Could you check a few things on this model? Use its own coordinates, in mm. Face numbers are marked on the shaded views. A direction names the side the tool comes from. Round coordinates to 2 decimals unless told otherwise and drop trailing zeros. Loops run counter-clockwise (first coordinate to the right, second up) from the corner with the lowest first, then second, coordinate; pieces in that order, holes last. Notation, with made-up numbers: M -25,-12.5 L -17,-12.5 A18 ccw -17,12.5 Z; hole C -25.5,79 d7. An arc over 180 degrees is marked long. Answer in a Markdown table with one row per item.
```python
from build123d import *

# Parameters (mm, degrees)
FILLET_1_R               = 4
CUT_EXTRUDE_3_DEPTH      = 6
PATTERN_CIRCULAR_2_COUNT = 6
SKETCH_5_W               = 18.3
SKETCH_5_H               = 8
CUT_EXTRUDE_4_DEPTH      = 20
SKETCH_6_R               = 6
CUT_EXTRUDE_5_DEPTH      = 146.688022843
SKETCH_7_R               = 6.6215
CUT_EXTRUDE_6_DEPTH      = 146.688022843


with BuildPart() as part:
    # Sketch 1 → Revolve 1 (revolve)
    with BuildSketch(Plane(origin=(0, 0, 0), x_dir=(1, 0, 0), z_dir=(0, 1, 0)), mode=Mode.PRIVATE) as revolve_1_sk:
        Polygon((15, 20), (30, 20), (30, 6), (70, 6), (70, 15), (100, 15), (100, -15), (70, -15), (70, -6), (30, -6), (30, -20), (15, -20), align=None)
    revolve(revolve_1_sk.sketch.rotate(Axis((0, 0, -20), (0, 0, 1)), 180), axis=Axis((0, 0, -20), (0, 0, 1)))

    # Fillet 1
    fillet_1_edges = [part.edges().sort_by_distance(p)[0] for p in [
        (30, 0, 6),
        (70, 0, 6),
        (70, 0, -6),
        (30, 0, -6),
    ]]
    fillet(fillet_1_edges, radius=FILLET_1_R)

    # Sketch 4 → Cut-Extrude 3 (cut, symmetric)
    with BuildSketch(Plane.XY):
        with BuildLine():
            Line((41.5692, 6), (55.9285, 6))
            ThreePointArc((55.9285, 6), (59.790137098, 7.823876746), (60.8345, 11.9649))
            ThreePointArc((60.8345, 11.9649), (53.693292616, 30.999275079), (40.779, 46.7004))
            ThreePointArc((40.779, 46.7004), (36.670623538, 47.866536224), (33.1603, 45.4342))
            Line((33.1603, 45.4342), (25.9807, 32.9996))
            ThreePointArc((25.9807, 32.9996), (25.354603735, 29.839289607), (26.7862, 26.9531))
            ThreePointArc((26.7862, 26.9531), (32.908684734, 18.999699449), (36.7356, 9.7209))
            ThreePointArc((36.7356, 9.7209), (38.519259186, 7.037974406), (41.5692, 6))
        make_face()
    cut_extrude_3 = extrude(amount=CUT_EXTRUDE_3_DEPTH, both=True, mode=Mode.SUBTRACT)

    # Pattern Circular 2: Cut-Extrude 3 ×6 about axis
    pattern_circular_2_axis = Axis((0, 0, 0), (0, 0, 1))
    for i in range(1, PATTERN_CIRCULAR_2_COUNT):
        add(cut_extrude_3.rotate(pattern_circular_2_axis, i * 360 / PATTERN_CIRCULAR_2_COUNT), mode=Mode.SUBTRACT)

    # Sketch 5 → Cut-Extrude 4 (cut, symmetric)
    with BuildSketch(Plane.XY):
        with Locations((9.15, 0)):
            Rectangle(SKETCH_5_W, SKETCH_5_H)
    extrude(amount=CUT_EXTRUDE_4_DEPTH, both=True, mode=Mode.SUBTRACT)

    # Sketch 6 → Cut-Extrude 5 (cut, through all)
    with BuildSketch(Plane.XY.offset(15)):
        with Locations((92, 0)):
            Circle(SKETCH_6_R)
    extrude(amount=-CUT_EXTRUDE_5_DEPTH, mode=Mode.SUBTRACT)

    # Sketch 7 → Cut-Extrude 6 (cut, through all)
    with BuildSketch(Plane.XY.offset(15)):
        with Locations((-80, 0)):
            Circle(SKETCH_7_R)
    extrude(amount=-CUT_EXTRUDE_6_DEPTH, mode=Mode.SUBTRACT)


solid = part.part
```
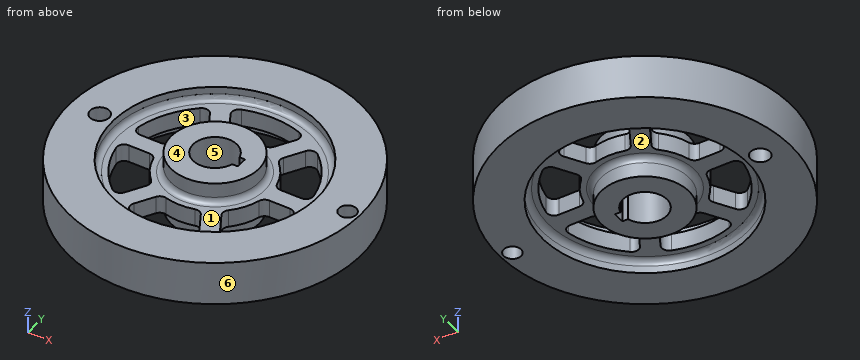
1) I want a section at A-A, the plane x = -80. Please give me the cut outline in (y, z).
Computed:
| item | result |
|---|---|
| outline | M -60,-15 L -6.62,-15 L -6.62,15 L -60,15 Z; M 6.62,-15 L 60,-15 L 60,15 L 6.62,15 Z |
2) Will these pins go through, and if not, where does the flat tip stop? P1, Ø3, axis at x = 16.5, z = -3, coming from the +Y side; P2, Ø3, axis at x = 15.5, z = -5.5, coming from the -Y side; P3, Ø12, axis at x = -43.5, z = 1, coming from the +Y side; P4, Ø12, axis at x = -75, y = -78, coming from the -Z side.
Computed:
| item | result |
|---|---|
| P1 | stops at y = 98.87 |
| P2 | stops at y = -99.02 |
| P3 | stops at y = 92.7 |
| P4 | passes through |
3) I want a section at D-D, the plane x = 92. Please give me the cut outline in (y, z), plus the area to 3 significant figures.
Computed:
| item | result |
|---|---|
| outline | M -39.19,-15 L -6,-15 L -6,15 L -39.19,15 Z; M 6,-15 L 39.19,-15 L 39.19,15 L 6,15 Z |
| area | 1,990 mm² |
4) Which directions (+Z, -Z, +X, -X, +Y, -Y) give clear straight access to the entire face, cutting with the end or side of a thin tool? Please do the marked faces 1, 2 and 3.
Computed:
| item | result |
|---|---|
| face 1 | +Z |
| face 2 | -Z |
| face 3 | +Z, -Z |
5) I need wall thicknesses on line 1 (Y direction, x = 0, z = -12); line 2 (Y direction, x = 0, z = -3); line 3 (X direction, y = 43, z = 4.5). Which ranges of each line are inside material? Lowest first, please.
Computed:
| item | result |
|---|---|
| line 1 | y = -100 to -70, -30 to -15, 15 to 30, 70 to 100 |
| line 2 | y = -100 to -62, -38 to -15, 15 to 38, 62 to 100 |
| line 3 | x = -90.28 to -44.67, -31.75 to -17.9, 17.9 to 31.75, 44.66 to 90.28 |
6) I want a section at B-B, the plane y = 0. State how many separate pieces and enclosed holes the cut face has, plus the area to 3 significant figures.
Computed:
| item | result |
|---|---|
| separate pieces | 4 |
| enclosed holes | 0 |
| area | 3,100 mm² |
7) If we mould it in two halves opening along Y, with no side actions, what happens to the marked faces 4, 5 and 6? For each: released by +Y, released by -Y, zero draft, split by the parting line, or undercut.
Computed:
| item | result |
|---|---|
| face 4 | zero draft |
| face 5 | undercut |
| face 6 | split by the parting line |
